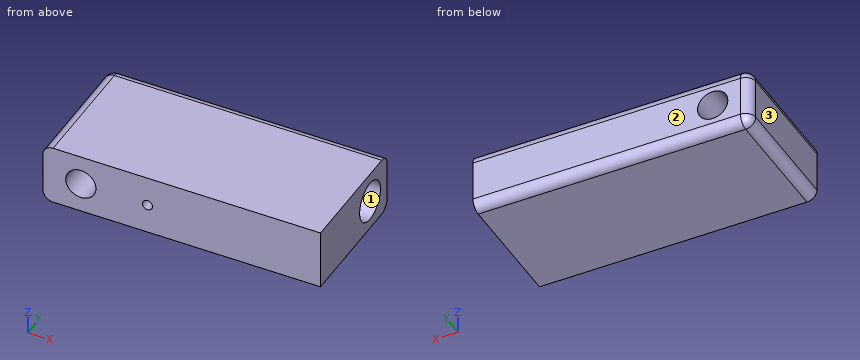
Autodesk Inventor part; units mm, degrees
ref_plane "YZ Plane" through (0, 0, 0) normal (1, 0, 0) x (0, 1, 0)
ref_plane "XZ Plane" through (0, 0, 0) normal (0, 1, 0) x (-1, 0, 0)
ref_plane "XY Plane" through (0, 0, 0) normal (0, 0, 1) x (1, 0, 0)
sketch "Esboço2" plane through (0, 0, 0) normal (0, 1, 0) x (-1, 0, 0)
  line L0 (0, 0) -> (-55, 0)
  line L1 (-55, 0) -> (-55, -12)
  line L2 (-55, -12) -> (0, -12)
  line L3 (0, -12) -> (0, 0)
  dimension "d0" = 55
  dimension "d1" = 12
extrude "Extrusão1" add sketch "Esboço2" along normal blind 25.5
sketch "Esboço3" plane through (0, 25.5, 0) normal (0, 1, 0) x (1, 0, 0)
  line L0 (0, 12) -> (0, 0)
  line L1 (0, 6) -> (7.5, 6)
  dimension "d4" = 7.5
hole "Furo1" at (7.5, 25.5, -6) direction (0, -1, 0) diameter 6 end through all
sketch "Esboço4" plane through (0, 0, 0) normal (0, -1, 0) x (1, 0, 0)
  circle A0 centre (7.5, -6) radius 3
  line L0 (7.5, -6) -> (20.7, -6)
  point P0 (0, 0)
  dimension "d12" = 13.2
sketch "Esboço5" plane through (55, 0, 0) normal (1, 0, 0) x (0, 0, -1)
  line L0 (0, 0) -> (0, 19)
  line L1 (0, 0) -> (0, 25.5)
  line L2 (0, 19) -> (6, 19)
  dimension "d13" = 19
  dimension "d14" = 6
hole "Furo2" at (55, 19, -6) direction (-1, 0, 0) diameter 8 depth 41
hole "Furo3" at (20.7, 0, -6) direction (0, 1, 0) diameter 2 depth 16
fillet "Arredondamento1" radius 2 5 edges at (0, 25.5, -6) (0, 12.75, 0) (0, 12.75, -12) (27.5, 25.5, 0) (27.5, 25.5, -12)
properties part number "cilinder"
Build history of the part. All positions in model axes, mm. Face numbers are marked on the shaded views. Round coordinates to 2 decimals unless told otherwise and drop trailing zeros. Loops run counter-clockwise (first coordinate to the right, second up) from the corner with the lowest first, then second, coordinate; pieces in that order, holes last. Notation, with made-up numbers: (-18.75, -22) -> (24.25, -22) arc R31 ccw to (24.25, 10) -> close; hole circle Ø11 at (2.25, 36.25). An arc over 180 degrees is marked (long way). One line per item, written item: value. Start each with the question number.
Q1. Two-plate mould, pull along Y, no slides. Class the marked faces 1, 2 and 3: released by +Y, released by -Y, zero draft, split by the parting line, or undercut.
Q2. Cut at D-D on x = 20.7. List the corners of the cut face in (y, z), plus the area to 3 significant figures.
Q3. Cut at B-B on z = -6. List the corners of the cut face in (x, y).
Q4. Probe line 1 along X through (y, z) = (14, -6); line 2 along Y through (x, z) = (24, -5.75); line 3 along Z through (x, y) = (20.7, 11). List the from-to ranges inside material, lowest first.
Q5. Drop flat-ended pins along their axis: pin 1 Ø6.5 at (y, z) = (19.5, -5.5) entering from +X; pin 2 Ø5.5 at (x, z) = (7.5, -6) entering from -Y. Give the stop position or say it passes through.
Q6. Cut at A-A on x = 7.5. List the corners of the cut face in (y, z), plus the area to 3 significant figures.
Q7. Cut at C-C on y = 19. List the corners of the cut face in (x, z).
Computed:
1. face 1: undercut
1. face 2: released by +Y
1. face 3: zero draft
2. outline: (0, -12) -> (23.5, -12) arc R2 ccw to (25.5, -10) -> (25.5, -2) arc R2 ccw to (23.5, 0) -> (0, 0) -> (0, -5) -> (15.13, -5) arc R4 cw (long way) to (15.13, -7) -> (0, -7) -> close
2. area: 224 mm²
3. outline: (0, 0) -> (4.5, 0) -> (4.5, 25.5) -> (2, 25.5) arc R2 ccw to (0, 23.5) -> close; (10.5, 0) -> (19.7, 0) -> (19.7, 15) -> (14, 15) -> (14, 23) -> (55, 23) -> (55, 25.5) -> (10.5, 25.5) -> close; (21.7, 0) -> (55, 0) -> (55, 15) -> (21.7, 15) -> close
4. line 1: 0 to 4.5, 10.5 to 19.7, 21.7 to 55
4. line 2: 0 to 15.01, 22.99 to 25.5
4. line 3: -12 to -7, -5 to 0
5. pin 1: x = 14
5. pin 2: through
6. outline: (0, -12) -> (23.5, -12) arc R2 ccw to (25.5, -10) -> (25.5, -9) -> (0, -9) -> close; (0, -3) -> (25.5, -3) -> (25.5, -2) arc R2 ccw to (23.5, 0) -> (0, 0) -> close
6. area: 151 mm²
7. outline: (0, -10) arc R2 ccw to (2, -12) -> (55, -12) -> (55, -10) -> (14, -10) -> (14, -2) -> (55, -2) -> (55, 0) -> (2, 0) arc R2 ccw to (0, -2) -> close; hole circle Ø6 at (7.5, -6)
